Part model, mm, in its own coordinate system. Face numbers are marked on the shaded views. A direction names the side the tool comes from. Round coordinates to 2 decimals unless told otherwise and drop trailing zeros. Write each loop counter-clockwise with the first axis right and the second up, starting at its lowest first coordinate (ties: lowest second). Pieces come first, ordered by that corner, then holes. Notation, with made-up numbers: M -24,28.5 L 14,28.5 A10 cw 14,42.5 Z; hole C 51.5,-33.75 d5. An arc over 180 degrees is marked long. Use a Markdown table: item, result. Add a question column.
1) Slice it at C-C on x = 0.5. Write the cut outline in (y, z) (3 decimals).
2) Slice it at A-A on z = 0. Write the cut outline in (x, y) (3 decimals), plus the area to 3 significant figures.
3) Two-plate mould, pull along Z, no slides. Class the marked faces 3, 4 and 5: released by +Z, released by -Z, zero draft, split by the parting line, or undercut.
4) Slice it at B-B on y = 0. Write the cut outline in (x, z) (3 decimals), plus the area to 3 significant figures.
5) Slice it at D-D on x = 2.15. Write the cut outline in (y, z) (3 decimals), plus the area to 3 significant figures.
6) Which spindle directions (+Z, -Z, +X, -X, +Y, -Y) get a long thin tool onto all of the face, cutting with end or side? Do the marked faces 1 and 2. Say none if no direction does.
7) Wall check: probe 1 along Z at (x, y) = (1.35, 0) (3 decimals); probe 2 along X at (y, z) = (-14, 3.5); probe 3 along Y at (x, z) = (1.95, 0) (3 decimals). Give the ranges that are in metal, low to high.
8) Drop flat-ended pins along their axis: P1, Ø1.8, axis at x = 4, y = -12, coming from the +Z side; P2, Ø2.5, axis at y = -13.5, z = 2, coming from the +X side; P3, Ø1.5, axis at x = 2, z = -1, coming from the -Y side. Give the stop position or say it passes through.
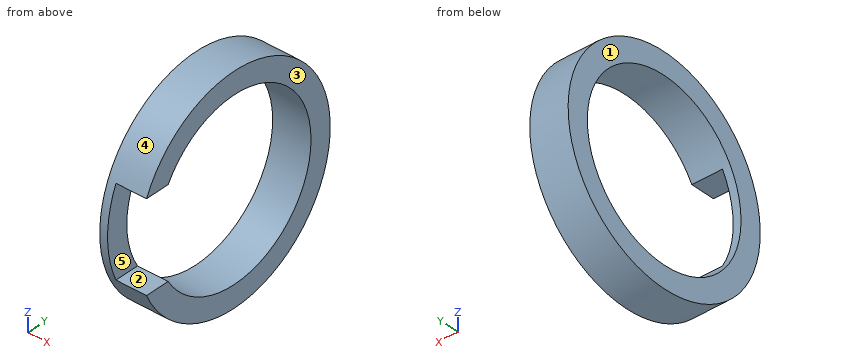
```python
from build123d import *

# Parameters (mm, degrees)
SKETCH1_R           = 15.875
SKETCH1_R_2         = 12.7
BOSS_EXTRUDE1_DEPTH = 5.588
CUT_EXTRUDE2_START  = -4.445
CUT_EXTRUDE2_DEPTH  = 4.445


with BuildPart() as part:
    # Sketch1 → Boss-Extrude1 (new body)
    with BuildSketch(Plane(origin=(0, 0, 0), x_dir=(0, 0, -1), z_dir=(1, 0, 0))):
        Circle(SKETCH1_R)
        Circle(SKETCH1_R_2, mode=Mode.SUBTRACT)
    extrude(amount=BOSS_EXTRUDE1_DEPTH)

    # Sketch3 → Cut-Extrude2 (cut)
    with BuildSketch(Plane(origin=(5.588, 0, 0), x_dir=(0, 0, -1), z_dir=(1, 0, 0)).offset(CUT_EXTRUDE2_START)):
        with BuildLine():
            Line((-6.477, -10.924214892), (-6.477, -14.4935881))
            ThreePointArc((-6.477, -14.4935881), (0, -15.875), (6.477, -14.4935881))
            Line((6.477, -14.4935881), (6.477, -10.924214892))
            Line((6.477, -10.924214892), (-6.477, -10.924214892))
        make_face()
    extrude(amount=CUT_EXTRUDE2_DEPTH, mode=Mode.SUBTRACT)


solid = part.part
```
Entries:
| question | item | result |
|---|---|---|
| 1 | outline | C 0,0 d31.75; hole C 0,0 d25.4 |
| 2 | outline | M 0,-15.875 L 1.143,-15.875 L 1.143,-12.7 L 0,-12.7 Z; M 0,12.7 L 5.588,12.7 L 5.588,15.875 L 0,15.875 Z |
| 2 | area | 21.4 mm^2 |
| 3 | face 3 | zero draft |
| 3 | face 4 | split by the parting line |
| 3 | face 5 | undercut |
| 4 | outline | M 0,-15.875 L 5.588,-15.875 L 5.588,-12.7 L 0,-12.7 Z; M 0,12.7 L 5.588,12.7 L 5.588,15.875 L 0,15.875 Z |
| 4 | area | 35.5 mm^2 |
| 5 | outline | M -14.494,-6.477 A15.875 ccw long -14.494,6.477 L -10.924,6.477 A12.7 cw long -10.924,-6.477 Z |
| 5 | area | 242 mm^2 |
| 6 | face 1 | +Z, -Z, -X, +Y, -Y |
| 6 | face 2 | +X, -Y |
| 7 | probe 1 | z = -15.875 to -12.7, 12.7 to 15.875 |
| 7 | probe 2 | x = 0 to 1.14 |
| 7 | probe 3 | y = 12.7 to 15.875 |
| 8 | P1 | stops at z = 11.35 |
| 8 | P2 | stops at x = 1.14 |
| 8 | P3 | stops at y = 12.58 |
